For this review, take the finished solid that the model builds, in its own axes (mm). A direction names the side the tool comes from. Give positions to 0.01 mm unless a question says otherwise; leave off trailing zeros. Loops run counter-clockwise (first coordinate to the right, second up) from the corner with the lowest first, then second, coordinate; pieces in that order, holes last. Notation, with made-up numbers: (-6, -40) -> (11, -40) arc R27 cw to (11, -19) -> close; hole circle Ø11 at (86.25, -37). An arc over 180 degrees is marked (long way). Answer as CSV lines item,"result". Start each with the question number.
Item 1: The part is to be moulded in two halves that separate along Z. For faces 1 (the face through (27, 0, -13)), 2 (the face through (3, -8, 4)), 3 (the face through (5, -30, -4)), 4 (the face through (20, 15, 8)), say which applies: +Z half, -Z half, draft (parallel to the pull), parting line (faces both ways), or undercut.
Item 2: For L1, parallel to Y at x = 25, z = -16.5; L2, parallel to Y at x = 25, z = 0; L3, parallel to Y at x = 17.5, z = -7, list the stretches that pass through material, from the lowest coordinate up. Write a range as from..to.
Item 3: Add section C-C on y = 0. State the section outline as (x, z) points, plus the area to 3 significant figures.
Item 4: Add section A-A on x = 26.5. State the section outline as (y, z) points, plus the area to 3 significant figures.
Item 5: Add section B-B on z = -20. State the section outline as (x, y) points, plus the area to 3 significant figures.
Item 6: Machinability: for faces 5 (the face through (25.07, 14.01, 6.74)), 6 (the face through (20, 6, -17)), 7 (the face through (19, -9, -21.9)), 8 (the face through (-1.73, -7.81, -0.06)), which of the approach directions +Z, -Z, +X, -X, +Y, -Y give a long, thin tool a straight path to every point of the face, cutting with its end or side? Answer none if there is none.
Item 7: Clearance check with flat-ended pins moving along their axes: P1, Ø3, axis at y = 14.5, z = 7, coming from the +X side; P2, Ø14.5, axis at x = 0, y = 0, coming from the -Z side; P3, Ø12, axis at x = 4, y = 1, coming from the -Z side; P4, Ø2.5, axis at x = 23.5, z = -19, coming from the +Y side. State where each tip first meets the part, or that it passes through.
```python
from build123d import *

# Parameters (mm, degrees)
SCHIZZO1_W                   = 60
SCHIZZO1_H                   = 60
SCHIZZO1_R                   = 8
ESTRUSIONE_ESTRUSIONE1_DEPTH = 4
SCHIZZO2_W                   = 60
SCHIZZO2_H                   = 60
SCHIZZO2_R                   = 12.1
ESTRUSIONE_ESTRUSIONE2_DEPTH = 8.5
SCHIZZO6_W                   = 60
SCHIZZO6_H                   = 60
SCHIZZO6_R                   = 12.1
ESTRUSIONE_ESTRUSIONE3_DEPTH = 9.4
SCHIZZO3_W                   = 60
SCHIZZO3_H                   = 10
TAGLIO_ESTRUSIONE1_DEPTH     = 55.620142805
RACCORDO2_R                  = 10
SCHIZZO10_R                  = 2.25
TAGLIO_ESTRUSIONE3_DEPTH     = 55.62014286
ESTRUSIONE_ESTRUSIONE5_DEPTH = 1
SMUSSO2_SIZE                 = 0.5
SCHIZZO12_R                  = 1.25
TAGLIO_ESTRUSIONE4_DEPTH     = 10
SCHIZZO14_W                  = 1.470153799
SCHIZZO14_H                  = 12
SCHIZZO14_W_2                = 1
SCHIZZO14_H_2                = 7
TAGLIO_ESTRUSIONE5_DEPTH     = 7
SMUSSO3_SIZE                 = 1


# Read off the part's stored shape, not the designer's step: Estrusione-Estrusione5
with BuildPart() as part:
    # Schizzo1 → Estrusione-Estrusione1 (new, symmetric)
    with BuildSketch(Plane.XY):
        Rectangle(SCHIZZO1_W, SCHIZZO1_H)
        Circle(SCHIZZO1_R, mode=Mode.SUBTRACT)
    extrude(amount=ESTRUSIONE_ESTRUSIONE1_DEPTH, both=True)

    # Schizzo2 → Estrusione-Estrusione2 (add)
    with BuildSketch(Plane.XY.offset(4)):
        Rectangle(SCHIZZO2_W, SCHIZZO2_H)
        Circle(SCHIZZO2_R, mode=Mode.SUBTRACT)
    estrusione_estrusione2 = extrude(amount=ESTRUSIONE_ESTRUSIONE2_DEPTH)

    # Specchia1: Estrusione-Estrusione2 across plane
    add(estrusione_estrusione2.mirror(Plane.XY))

    # Schizzo6 → Estrusione-Estrusione3 (add)
    with BuildSketch(Plane(origin=(0, 0, -12.5), x_dir=(-1, 0, 0), z_dir=(0, 0, -1))):
        Rectangle(SCHIZZO6_W, SCHIZZO6_H)
        with Locations(Location((0, 0, 0), (0, 0, 180))):
            Circle(SCHIZZO6_R, mode=Mode.SUBTRACT)
    extrude(amount=ESTRUSIONE_ESTRUSIONE3_DEPTH)

    # Schizzo3 → Taglio-Estrusione1 (cut, through all)
    with BuildSketch(Plane.XY.offset(12.5)):
        with Locations((0, 25)):
            Rectangle(SCHIZZO3_W, SCHIZZO3_H)
    extrude(amount=-TAGLIO_ESTRUSIONE1_DEPTH, mode=Mode.SUBTRACT)

    # Raccordo2
    raccordo2_edges = [part.edges().sort_by_distance(p)[0] for p in [
        (-30, -30, -4.7),
    ]]
    fillet(raccordo2_edges, radius=RACCORDO2_R)

    # Schizzo13 → Taglia-Rivoluzione4 (revolve, cut)
    with BuildSketch(Plane(origin=(0, 0, -30.4), x_dir=(-1, 0, 0), z_dir=(0, 0, -1))):
        Polygon((-9.5, 25.081325019), (-22, 25.081325019), (-22, -19), (2, -19), (2, -12), (-16, -12), (-16, -6), (-5.6, -6), (-5.6, 6), (-11, 6), (-11, 12), (-9.5, 12), align=None)
    revolve(axis=Axis((23, 27.323096352, -30.4), (0, -1, 0)), mode=Mode.SUBTRACT)

    # Schizzo10 → Taglio-Estrusione3 (cut, through all)
    with BuildSketch(Plane(origin=(0, 0, -21.9), x_dir=(-1, 0, 0), z_dir=(0, 0, -1))):
        with Locations((-25, -25)):
            Circle(SCHIZZO10_R)
        with Locations((22.656854249, -22.656854249)):
            Circle(SCHIZZO10_R)
        with Locations((25, 15)):
            Circle(SCHIZZO10_R)
    extrude(amount=-TAGLIO_ESTRUSIONE3_DEPTH, mode=Mode.SUBTRACT)

    # Estrusione-Estrusione5 outline → Estrusione-Estrusione5 (add)
    with BuildSketch(Plane(origin=(0, 0, -21.9), x_dir=(-1, 0, 0), z_dir=(0, 0, -1))):
        with BuildLine():
            Line((14, 19.9), (14, 18.9))
            ThreePointArc((14, 18.9), (17.464823228, 17.464823228), (18.9, 14))
            Line((18.9, 14), (18.9, -14))
            ThreePointArc((18.9, -14), (17.464823228, -17.464823228), (14, -18.9))
            Line((14, -18.9), (0.510635891, -18.9))
            Line((0.510635891, -18.9), (0.510635891, -19))
            Line((0.510635891, -19), (-30, -19))
            Line((-30, -19), (-30, -19.9))
            Line((-30, -19.9), (14, -19.9))
            ThreePointArc((14, -19.9), (18.171930009, -18.171930009), (19.9, -14))
            Line((19.9, -14), (19.9, 14))
            ThreePointArc((19.9, 14), (18.171930009, 18.171930009), (14, 19.9))
        make_face()
    extrude(amount=ESTRUSIONE_ESTRUSIONE5_DEPTH)

    # Smusso2
    smusso2_edges = [part.edges().sort_by_distance(p)[0] for p in [
        (8, -19.9, -22.9),
        (-18.171930009, -18.171930009, -22.9),
        (-19.9, 0, -22.9),
        (-18.171930009, 18.171930009, -22.9),
    ]]
    chamfer(smusso2_edges, length=SMUSSO2_SIZE)

    # Schizzo12 → Taglio-Estrusione4 (cut)
    with BuildSketch(Plane(origin=(30, 0, 0), x_dir=(0, 0, -1), z_dir=(1, 0, 0))):
        with Locations(Location((-7.5, -15, 0), (0, 0, 90))):
            Circle(SCHIZZO12_R)
        with Locations(Location((-7.5, 15, 0), (0, 0, 90))):
            Circle(SCHIZZO12_R)
    extrude(amount=-TAGLIO_ESTRUSIONE4_DEPTH, mode=Mode.SUBTRACT)

    # Schizzo14 → Taglio-Estrusione5 (cut)
    with BuildSketch(Plane(origin=(30, 0, 0), x_dir=(0, 0, -1), z_dir=(1, 0, 0))):
        with Locations((13.7350769, 0)):
            Rectangle(SCHIZZO14_W, SCHIZZO14_H)
        Polygon((20.653205655, 6), (20.653205655, 12), (18.856603619, 12), (18.856603619, 20), (16.9, 20), (16.9, 12), (18.4, 12), (18.4, 6), align=None)
        with Locations((5.9, -15.5)):
            Rectangle(SCHIZZO14_W_2, SCHIZZO14_H_2)
    extrude(amount=-TAGLIO_ESTRUSIONE5_DEPTH, mode=Mode.SUBTRACT)

    # Smusso3
    smusso3_edges = [part.edges().sort_by_distance(p)[0] for p in [
        (-12.1, 0, 12.5),
    ]]
    chamfer(smusso3_edges, length=SMUSSO3_SIZE)


solid = part.part
```
Computed values:
1,face 1,"-Z half"
1,face 2,"+Z half"
1,face 3,"draft"
1,face 4,"undercut"
2,L1,"-30..-27.25, -22.75..-19, -12..-6, 6..20"
2,L2,"-30..-27.25, -22.75..20"
2,L3,"-30..-19, -12..20"
3,outline,"(-30, -21.9) -> (-19.9, -21.9) -> (-19.9, -22.4) -> (-19.4, -22.9) -> (-18.9, -22.9) -> (-18.9, -21.9) -> (-12.1, -21.9) -> (-12.1, -4) -> (-8, -4) -> (-8, 4) -> (-12.1, 4) -> (-12.1, 11.5) -> (-13.1, 12.5) -> (-30, 12.5) -> close; (8, -4) -> (12.1, -4) -> (12.1, -16.84) arc R17.4 cw to (23, -13) -> (30, -13) -> (30, 12.5) -> (13.1, 12.5) -> (12.1, 11.5) -> (12.1, 4) -> (8, 4) -> close"
3,area,"1,150 mm²"
4,outline,"(-30, -21.9) -> (-26.68, -21.9) -> (-26.68, 12.5) -> (-30, 12.5) -> close; (-23.32, -21.9) -> (-19.9, -21.9) -> (-19.9, -22.4) -> (-19.4, -22.9) -> (-19, -22.9) -> (-19, -5.4) -> (-12, -5.4) -> (-12, -21.9) -> (-6, -21.9) -> (-6, -13) -> (6, -13) -> (6, -18.4) -> (12, -18.4) -> (12, -16.9) -> (20, -16.9) -> (20, 12.5) -> (-23.32, 12.5) -> close; hole circle Ø2.5 at (-15, 7.5); hole circle Ø2.5 at (15, 7.5)"
4,area,"1,310 mm²"
5,outline,"(-30, -20) arc R10 ccw to (-20, -30) -> (30, -30) -> (30, -19) -> (0.27, -19) -> (0.27, -12.1) arc R12.1 cw (long way) to (10.51, 6) -> (17.01, 6) -> (17.01, 12) -> (14.39, 12) -> (14.39, 20) -> (-30, 20) -> close; (1.55, -12) -> (30, -12) -> (30, -6) -> (10.51, -6) arc R12.1 cw to start; hole circle Ø4.5 at (-25, 15); hole circle Ø4.5 at (-22.66, -22.66); hole circle Ø4.5 at (25, -25)"
5,area,"1,840 mm²"
6,face 5,"+X"
6,face 6,"-Z, +X"
6,face 7,"-Z, +X, +Y"
6,face 8,"+Z, -Z"
7,P1,"x = 30"
7,P2,"through"
7,P3,"z = -4"
7,P4,"y = 12"
